Here's how the part is built. I have some questions about the finished solid (model axes, mm). Round coordinates to 2 decimals unless told otherwise and drop trailing zeros. Loops run counter-clockwise (first coordinate to the right, second up) from the corner with the lowest first, then second, coordinate; pieces in that order, holes last. Notation, with made-up numbers: M 0.25,-16.75 L 23.25,-16.75 A20 cw 23.25,-2.75 Z; hole C 20,36 d6. An arc over 180 degrees is marked long. Put each result on its own line as item: value. Start each with the question number.
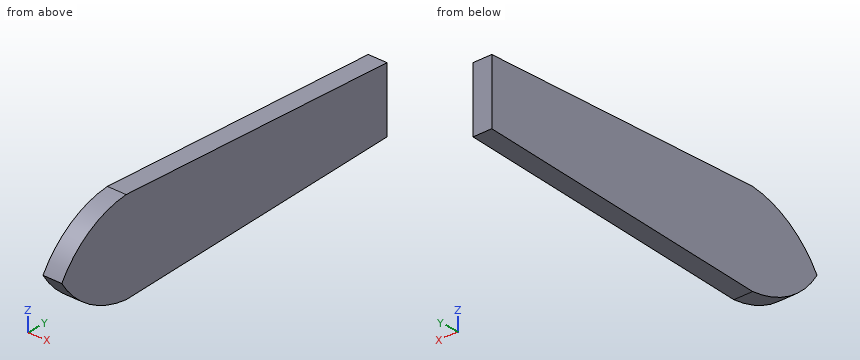
```python
from build123d import *

# Parameters (mm, degrees)
F1_DEPTH = 6.858


# Not quite as in the source:
# - the program builds the solid bodies; features that only make, move or delete a surface that nothing else refers to are left out


with BuildPart() as f1:
    # F0 (on Right) → F1 (new body)
    with BuildSketch(Plane.YZ):
        with BuildLine():
            Line((61.0633231699, 11.7456540465), (-47.3298765719, 16.6299846023))
            ThreePointArc((-47.3298765719, 16.6299846023), (-62.6691287871, 11.4749888817), (-74.0792676806, 0))
            Line((-74.0792676806, 0), (61.0633231699, 0))
            Line((61.0633231699, 0), (61.0633231699, 11.7456540465))
        make_face()
        with BuildLine():
            Line((61.0633231699, 0), (-74.0792676806, 0))
            ThreePointArc((-74.0792676806, 0), (-62.6691287871, -11.4749888817), (-47.3298765719, -16.6299846023))
            Line((-47.3298765719, -16.6299846023), (61.0633231699, -11.7456540465))
            Line((61.0633231699, -11.7456540465), (61.0633231699, 0))
        make_face()
    extrude(amount=F1_DEPTH)


solid = f1.part
```
1) Suppose I cut it at A-A (x = 3). Write out the boundary of the cut face in (y, z).
2) Suppose I cut it at C-C (y = 5). Write out the boundary of the cut face in (x, z), plus the area to 3 significant figures.
3) If I drill on probe 1 along Z at (x, y) = (4.5, -19.5); probe 2 along Z at (x, y) = (3.75, 20.5); probe 3 along Y at (x, z) = (0.5, -3), over which ranges is the centre line in solid material (lowest first)? Write a range as from..to.
4) I'm going to push flat-ended pins straight in: P1, Ø2, axis at x = 4.5, z = 10, coming from the -Y side; P2, Ø2, axis at x = 6, z = -11, coming from the -Y side; P3, Ø4, axis at x = 1.5, y = -28.5, coming from the -Z side. Where does each tip first touch, or does it pass through?
5) Suppose I cut it at B-B (z = 15.5). Write out the boundary of the cut face in (x, y).
Results are:
1. outline: M -74.08,0 A35.19 ccw -47.33,-16.63 L 61.06,-11.75 L 61.06,11.75 L -47.33,16.63 A35.19 ccw Z
2. outline: M 0,-14.27 L 6.86,-14.27 L 6.86,14.27 L 0,14.27 Z
2. area: 196 mm²
3. probe 1: -15.38..15.38
3. probe 2: -13.57..13.57
3. probe 3: -72.02..61.06
4. P1: y = -66.16
4. P2: y = -64.85
4. P3: z = -15.87
5. outline: M 0,-53.49 L 6.86,-53.49 L 6.86,-22.25 L 0,-22.25 Z
